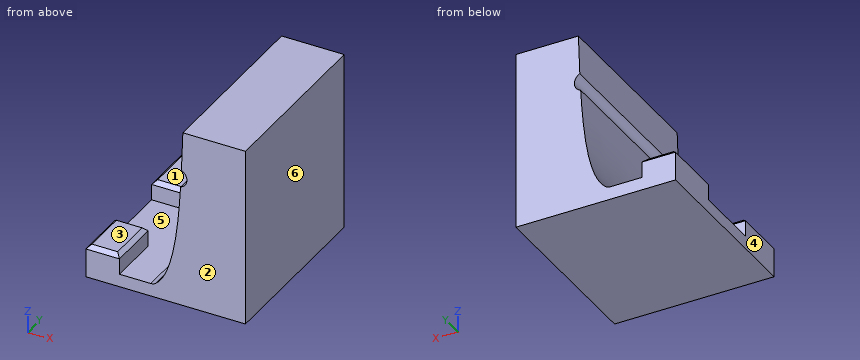
from build123d import *

# Parameters (mm, degrees)
F7_DEPTH = 114.3
F0_W     = 21.425565113
F0_H     = 33.2948663116
F8_DEPTH = 12.7
F0_H_2   = 38.15253824
F9_DEPTH = 12.7
F10_SIZE = 2.54
F1_SIZE  = 2.54
F11_SIZE = 2.54
F2_SIZE  = 2.54
F12_SIZE = 2.54
F3_SIZE  = 2.54
F4_SIZE  = 2.54
F13_R    = 5.08


# Not quite as in the source:
# - a feature of the source that left no trace in its solid (it failed there, or was rolled back) is left out


with BuildPart() as f7:
    # F6 (on Front) → F7 (new body)
    with BuildSketch(Plane.XZ):
        with BuildLine():
            Line((28.0298027718, 88.895993849), (-11.7995445112, 88.895993849))
            add(Edge.make_bspline(
                [(-12.7191172273, 63.6731384112), (-12.3630729131, 71.9399928392), (-12.0813087773, 80.417993931), (-11.7995445112, 88.895993849)],
                knots=[0.894750445, 0.894750445, 0.894750445, 0.894750445, 1, 1, 1, 1], degree=3))
            ThreePointArc((-12.7191172273, 63.6731384112), (-9.233937312, 57.9257119158), (-13.2581382148, 52.5419216657))
            add(Edge.make_bspline(
                [(-30.7190670022, -17.1741323863), (-19.0091812538, -10.6770336575), (-15.1403430342, 18.1088676273), (-13.2581382148, 52.5419216657)],
                knots=[0.3956141416, 0.3956141416, 0.3956141416, 0.3956141416, 0.846870688, 0.846870688, 0.846870688, 0.846870688], degree=3))
            add(Edge.make_bspline(
                [(-44.7375965866, -17.1741323863), (-39.4125863388, -19.0279691828), (-34.6287794117, -19.3433924519), (-30.7190670022, -17.1741323863)],
                knots=[0.2449479988, 0.2449479988, 0.2449479988, 0.2449479988, 0.3956141416, 0.3956141416, 0.3956141416, 0.3956141416], degree=3))
            Line((-44.7375965866, -17.1741323863), (-49.7875006466, -17.1741323863))
            Line((-49.7875006466, -17.1741323863), (-73.5701972282, -17.1741323863))
            Line((-73.5701972282, -17.1741323863), (-73.5701972282, -25.404006151))
            Line((-73.5701972282, -25.404006151), (28.0298027718, -25.404006151))
            Line((28.0298027718, -25.404006151), (28.0298027718, 88.895993849))
        make_face()
        with BuildLine():
            add(Edge.make_bspline(
                [(-44.7375965866, -17.1741323863), (-39.4125863388, -19.0279691828), (-34.6287794117, -19.3433924519), (-30.7190670022, -17.1741323863)],
                knots=[0.2449479988, 0.2449479988, 0.2449479988, 0.2449479988, 0.3956141416, 0.3956141416, 0.3956141416, 0.3956141416], degree=3))
            Line((-30.7190670022, -17.1741323863), (-44.7375965866, -17.1741323863))
        make_face()
    extrude(amount=F7_DEPTH)

    # F0 (on face) → F8 (join)
    with BuildSketch(Plane.XY.offset(-17.1741323863)):
        with Locations((-62.8574146717, -97.6525668442)):
            Rectangle(F0_W, F0_H)
    extrude(amount=F8_DEPTH)

    # F0 (on face) → F9 (join)
    with BuildSketch(Plane.XY.offset(-17.1741323863)):
        with Locations((-62.8574146717, -19.07626912)):
            Rectangle(F0_W, F0_H_2)
    extrude(amount=F9_DEPTH)

    # F10
    f10_edges = [f7.edges().sort_by_distance(p)[0] for p in [
        (-62.857415, 0, -4.474132),
    ]]
    chamfer(f10_edges, length=F10_SIZE)

    # F1
    f1_edges = [f7.edges().sort_by_distance(p)[0] for p in [
        (-52.144632, -20.346269, -4.474132),
        (-52.144632, -97.652567, -4.474132),
    ]]
    chamfer(f1_edges, length=F1_SIZE)

    # F11
    f11_edges = [f7.edges().sort_by_distance(p)[0] for p in [
        (-73.570197, -20.346269, -4.474132),
    ]]
    chamfer(f11_edges, length=F11_SIZE)

    # F2
    f2_edges = [f7.edges().sort_by_distance(p)[0] for p in [
        (-62.857415, -38.152538, -4.474132),
    ]]
    chamfer(f2_edges, length=F2_SIZE)

    # F12
    f12_edges = [f7.edges().sort_by_distance(p)[0] for p in [
        (-64.127415, -114.3, -4.474132),
    ]]
    chamfer(f12_edges, length=F12_SIZE)

    # F3
    f3_edges = [f7.edges().sort_by_distance(p)[0] for p in [
        (-73.570197, -96.382567, -4.474132),
    ]]
    chamfer(f3_edges, length=F3_SIZE)

    # F4
    f4_edges = [f7.edges().sort_by_distance(p)[0] for p in [
        (-62.857415, -81.005134, -4.474132),
    ]]
    chamfer(f4_edges, length=F4_SIZE)

    # F13
    f13_edges = [f7.edges().sort_by_distance(p)[0] for p in [
        (-30.719067, -57.15, -17.174132),
    ]]
    fillet(f13_edges, radius=F13_R)


solid = f7.part
CAD build for the part. Positions are in the model's coordinates, mm. Face numbers are marked on the shaded views. A direction names the side the tool comes from. Coordinates: 2 decimals unless noted, no trailing zeros. Loops run counter-clockwise (first coordinate to the right, second up) from the corner with the lowest first, then second, coordinate; pieces in that order, holes last. Notation, with made-up numbers: (77, 80.5) - (122, 80.5) arc R16 cw to (122, 98.5) - close; hole circle Ø8 at (-27.75, -22.75). An arc over 180 degrees is marked (long way). Write item = value, one per line. Start each with the question number.
Q1. Drill centre lines: L1, parallel to Z at x = -33.5, y = -91; L2, parallel to X at y = -88.5, z = -16.5; L3, parallel to Z at x = -57, y = -103. Where is each one in solid material? Low to high.
Q2. Cut at B-B, the plane x = -41.5. List the corners of the cut face in (y, z), then the cut area to 3 significant figures.
Q3. Pull direction X, two halves, no side cores. Call the marked faces 3, 4, 5 and 6: pulls with the +X half, pulls with the -X half, needs draft (parallel to the pull), parting line crosses it, or undercut.
Q4. Flat gauge pins, fed straight in: pin 1 Ø5 at (x, z) = (-64.5, -12.5) entering from +Y; pin 2 Ø5 at (x, y) = (-66.5, -101) entering from +Z; pin 3 Ø1 at (y, z) = (-92, 11.5) entering from -X. Where does each tip first touch, or does it go through?
Q5. Which spindle directions (+Z, -Z, +X, -X, +Y, -Y) get a long thin tool onto all of the face, cutting with end or side? Do the marked faces 1 and 2. Say none if no direction does.
Q6. Cut at A-A, the plane z = -12.5. Give the number of separate pieces and of enclosed holes in the cut face, then the cut area to 3 significant figures.
Computed:
q1.L1 = -25.4 to -17.17
q1.L2 = -73.57 to -52.14, -29.7 to 28.03
q1.L3 = -25.4 to -4.47
q2.outline = (-114.3, -25.4) - (0, -25.4) - (0, -17.17) - (-114.3, -17.17) - close
q2.area = 941 mm²
q3.face_3 = needs draft
q3.face_4 = pulls with the -X half
q3.face_5 = undercut
q3.face_6 = pulls with the +X half
q4.pin_1 = 0
q4.pin_2 = -4.47
q4.pin_3 = -17.54
q5.face_1 = +Z, -X, +Y, -Y
q5.face_2 = +Z, -Z, +X, -X, -Y
q6.separate_pieces = 3
q6.enclosed_holes = 0
q6.area = 7,680 mm²
